Geometry check sheet. Reference: the model listing, model coordinates, mm. A direction names the side the tool comes from. Give positions to 0.01 mm unless a question says otherwise; leave off trailing zeros. Write each loop counter-clockwise with the first axis right and the second up, starting at its lowest first coordinate (ties: lowest second). Pieces come first, ordered by that corner, then holes. Notation, with made-up numbers: (0, -0.5) - (9, -0.5) arc R19 cw to (9, 8.5) - close; hole circle Ø7 at (-35, -20.5). An arc over 180 degrees is marked (long way). Use a Markdown table: item, result.
```python
from build123d import *

# Parameters (mm, degrees)
PAD_DEPTH    = 220
SKETCH002_R  = 2
POCKET_DEPTH = 5.5
FILLET_R     = 2
FILLET001_R  = 1


with BuildPart() as part:
    # Sketch → Pad (new body)
    with BuildSketch(Plane.XZ):
        Polygon((-95, 0.548531), (-95, 3.548531), (95, 3.548531), (95, 0.548531), (110, 0.548531), (110, 7.548531), (-110, 7.548531), (-110, 0.548531), align=None)
    extrude(amount=PAD_DEPTH)

    # Sketch002 (on DatumPlane) → Pocket (cut, symmetric)
    with BuildSketch(Plane.XY.offset(6)):
        with Locations((-24.3, -113.85)):
            Circle(SKETCH002_R)
        with Locations((-24.3, -102.15)):
            Circle(SKETCH002_R)
    pocket = extrude(amount=POCKET_DEPTH, both=True, mode=Mode.SUBTRACT)

    # Mirrored: Pocket across Sketch002 V_Axis
    add(pocket.mirror(Plane(origin=(0, 0, 6), x_dir=(0, 0, 1), z_dir=(1, 0, 0))), mode=Mode.SUBTRACT)

    # Fillet
    fillet_edges = [part.edges().sort_by_distance(p)[0] for p in [
        (0, 0, 7.548531),
        (-110, -110, 7.548531),
        (0, -220, 7.548531),
        (110, -110, 7.548531),
    ]]
    fillet(fillet_edges, radius=FILLET_R)

    # Fillet001
    fillet001_edges = [part.edges().sort_by_distance(p)[0] for p in [
        (-26.3, -113.85, 3.548531),
        (-26.3, -102.15, 3.548531),
        (26.3, -113.85, 3.548531),
        (26.3, -102.15, 3.548531),
    ]]
    fillet(fillet001_edges, radius=FILLET001_R)


solid = part.part
```
1) Material ranges on L1, parallel to Y at x = 24.3, z = 5; L2, parallel to X at y = -16, z = 2.75; L3, parallel to Y at x = 24.3, z = 7.25, recorded low to high. Write a range as from..to.
Working result:
| item | result |
|---|---|
| L1 | y = -220..-115.85, -111.85..-104.15, -100.15..0 |
| L2 | x = -110..-95, 95..110 |
| L3 | y = -219.05..-115.85, -111.85..-104.15, -100.15..-0.95 |
2) Depth check by flat-ended pin: P1, Ø4.5, axis at x = 24.3, y = -102.15, coming from the -Z side; P2, Ø3.5, axis at x = 24.3, y = -113.85, coming from the -Z side. Enter the tip coordinate at first touch or a pass-through.
Working result:
| item | result |
|---|---|
| P1 | stops at z = 3.89 |
| P2 | passes through |
3) Set-up check for faces 1 (the flat face through (-1, -108, 3.549)), 2 (the flat face through (2, -108, 7.549)): record each of +Z, -Z, +X, -X, +Y, -Y from which the full face is reachable in a straight line by a thin tool's end or side.
Working result:
| item | result |
|---|---|
| face 1 | -Z, +Y, -Y |
| face 2 | +Z, +X, -X, +Y, -Y |
4) Section check A-A on z = 2.25. Record the boundary of the cut face in (x, y), then the cut area to 3 significant figures.
Working result:
| item | result |
|---|---|
| outline | (-110, -220) - (-95, -220) - (-95, 0) - (-110, 0) - close; (95, -220) - (110, -220) - (110, 0) - (95, 0) - close |
| area | 6,600 mm² |
5) Section check B-B on y = -122.5. Record the boundary of the cut face in (x, z), then the cut area to 3 significant figures.
Working result:
| item | result |
|---|---|
| outline | (-110, 0.55) - (-95, 0.55) - (-95, 3.55) - (95, 3.55) - (95, 0.55) - (110, 0.55) - (110, 5.55) arc R2 ccw to (108, 7.55) - (-108, 7.55) arc R2 ccw to (-110, 5.55) - close |
| area | 968 mm² |
6) Section check C-C on x = -58.5. Record the boundary of the cut face in (y, z).
Working result:
| item | result |
|---|---|
| outline | (-220, 3.55) - (0, 3.55) - (0, 5.55) arc R2 ccw to (-2, 7.55) - (-218, 7.55) arc R2 ccw to (-220, 5.55) - close |
